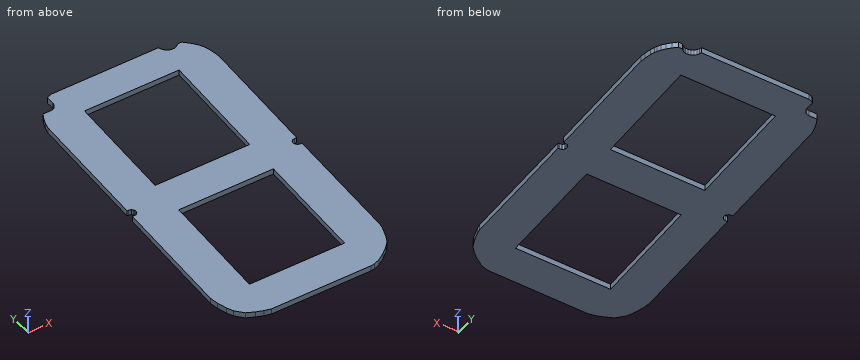
```python
from build123d import *

# Parameters (mm, degrees)
AUFSATZ_LINEAR_AUSTRAGEN1_DEPTH = 1.6


with BuildPart() as part:
    # Skizze1 → Aufsatz-Linear austragen1 (new body)
    with BuildSketch(Plane.XY):
        Polygon((17.145, -47.307483333), (19.05, -45.720016667), (20.478733333, -44.132516667), (21.431266667, -42.227516667), (22.5425, -39.21125), (22.86, -37.782483333), (25.0825, -0.79375), (24.60625, -0.79375), (23.97125, -0.635), (23.495, -0.15875), (23.33625, 0.47625), (23.495, 1.11125), (23.97125, 1.5875), (24.60625, 1.74625), (25.24125, 1.74625), (27.6225, 38.57625), (27.463733333, 40.004983333), (27.146266667, 42.06875), (26.828733333, 43.180016667), (26.511266667, 43.97375), (26.035, 44.92625), (25.241266667, 46.037516667), (24.288766667, 47.14875), (23.1775, 48.259983333), (21.9075, 48.259983333), (21.431266667, 47.78375), (20.955, 47.46625), (20.32, 47.307516667), (19.685, 47.307516667), (18.891266667, 47.46625), (18.256266667, 47.942516667), (17.78, 48.41875), (17.4625, 49.05375), (17.303733333, 49.68875), (12.7, 49.68875), (-14.605, 49.68875), (-15.5575, 49.37125), (-16.1925, 49.05375), (-16.1925, 46.83125), (-16.351266667, 46.037516667), (-16.668733333, 45.402516667), (-16.986266667, 44.92625), (-17.4625, 44.60875), (-18.256266667, 44.450016667), (-20.6375, 44.450016667), (-21.431266667, 43.02125), (-22.225, 41.11625), (-22.701266667, 39.21125), (-25.0825, 1.74625), (-24.606266667, 1.74625), (-23.971266667, 1.587516667), (-23.495, 1.11125), (-23.336266667, 0.47625), (-23.495, -0.15875), (-23.971266667, -0.635016667), (-24.606266667, -0.79375), (-25.247066667, -0.793383333), (-27.6225, -37.782483333), (-27.305, -40.322483333), (-26.511266667, -43.180016667), (-25.7175, -45.085016667), (-23.8125, -47.307483333), (-21.59, -48.41875), (-19.526266667, -49.212483333), (-17.621266667, -49.68875), (11.906266667, -49.68875), (13.0175, -49.530016667), (14.763733333, -48.895016667), align=None)
        Polygon((13.6525, -5.080016667), (-14.446266667, -5.080016667), (-16.668733333, -38.735016667), (11.588733333, -38.735016667), align=None, mode=Mode.SUBTRACT)
        Polygon((-13.811266667, 6.032516667), (-11.588733333, 39.687516667), (16.51, 39.687516667), (14.2875, 6.032516667), align=None, mode=Mode.SUBTRACT)
    extrude(amount=AUFSATZ_LINEAR_AUSTRAGEN1_DEPTH)


solid = part.part
```
Geometry check sheet. Reference: the model listing, model coordinates, mm. Give positions to 0.01 mm unless a question says otherwise; leave off trailing zeros. Write each loop counter-clockwise with the first axis right and the second up, starting at its lowest first coordinate (ties: lowest second). Pieces come first, ordered by that corner, then holes.
1) Section check B-B, the plane y = -16.5. Record the boundary of the cut face in (x, z), and give its area (3 significant figures).
2) Gauge pin test, flat ends, axial feed: pin 1 (0.5 mm diameter, centred on x = -19, z = 0.5, fed in from +Y); pin 2 (0.5 mm diameter, centred on x = 25, z = 1, fed in from +Y); pin 3 (0.5 mm diameter, centred on y = 47.5, z = 0.5, fed in from -X); pin 4 (5 mm diameter, centred on x = -11, y = -24, fed in from +Z). Record the tip position at first contact, or that the pin passes through.
3) Section check A-A, the plane x = -1.5. Record the boundary of the cut face in (y, z).
4) Section check D-D, the plane y = 28.5. Record the boundary of the cut face in (x, z), and give its area (3 significant figures).
5) Material ranges on L1, parallel to Y at x = -10, z = 0.75; L2, parallel to X at y = 18.5, z = 0.25; L3, parallel to Y at x = -14, z = 0.3, recorded low to high.
6) Section check C-C, the plane z = 1. State how many separate pieces and enclosed holes the cut face has, and give its area (3 significant figures).
Computed:
1. outline: (-26.26, 0) - (-15.2, 0) - (-15.2, 1.6) - (-26.26, 1.6) - close; (12.95, 0) - (24.14, 0) - (24.14, 1.6) - (12.95, 1.6) - close
1. area: 35.6 mm2
2. pin 1: stops at y = 44.45
2. pin 2: stops at y = 46.61
2. pin 3: stops at x = -16.19
2. pin 4: passes through
3. outline: (-49.69, 0) - (-38.74, 0) - (-38.74, 1.6) - (-49.69, 1.6) - close; (-5.08, 0) - (6.03, 0) - (6.03, 1.6) - (-5.08, 1.6) - close; (39.69, 0) - (49.69, 0) - (49.69, 1.6) - (39.69, 1.6) - close
4. outline: (-23.38, 0) - (-12.33, 0) - (-12.33, 1.6) - (-23.38, 1.6) - close; (15.77, 0) - (26.97, 0) - (26.97, 1.6) - (15.77, 1.6) - close
4. area: 35.6 mm2
5. L1: y = -49.69 to -38.74, -5.08 to 6.03, 39.69 to 49.69
5. L2: x = -24.02 to -12.99, 15.11 to 26.32
5. L3: y = -49.69 to -38.74, -5.08 to 49.69
6. separate pieces: 1
6. enclosed holes: 2
6. area: 2,970 mm2
